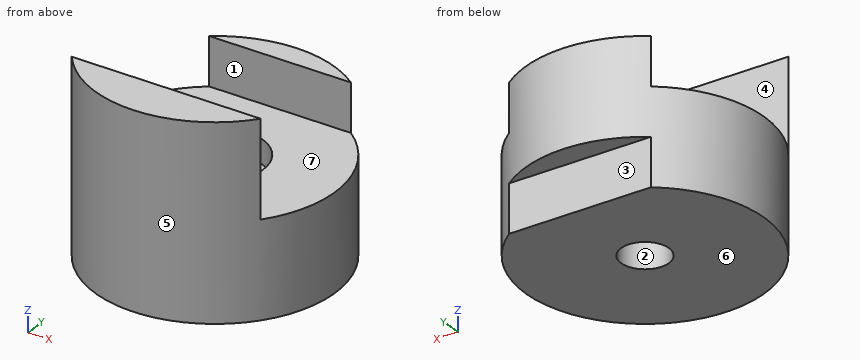
```python
from build123d import *

# Parameters (mm, degrees)
SKETCH1_R           = 5
SKETCH1_R_2         = 1
BOSS_EXTRUDE1_DEPTH = 8
SKETCH2_W           = 2
SKETCH2_H           = 1
CUT_EXTRUDE1_DEPTH  = 9
SKETCH3_R           = 2
CUT_EXTRUDE2_DEPTH  = 1


with BuildPart() as part:
    # Sketch1 → Boss-Extrude1 (new body)
    with BuildSketch(Plane.XY):
        Circle(SKETCH1_R)
        Circle(SKETCH1_R_2, mode=Mode.SUBTRACT)
    extrude(amount=BOSS_EXTRUDE1_DEPTH)

    # Sketch2 → Cut-Extrude1 (cut, symmetric)
    with BuildSketch(Plane(origin=(0, 0, 0), x_dir=(0, 0, -1), z_dir=(1, 0, 0))):
        Polygon((-8, -3), (-4, -3), (-4, 4), (-6, 4), (-6, 5), (-8, 5), align=None)
        with Locations((-1, 4.5)):
            Rectangle(SKETCH2_W, SKETCH2_H)
    extrude(amount=CUT_EXTRUDE1_DEPTH, both=True, mode=Mode.SUBTRACT)

    # Sketch3 → Cut-Extrude2 (cut)
    with BuildSketch(Plane.XY.offset(4)):
        Circle(SKETCH3_R)
    extrude(amount=-CUT_EXTRUDE2_DEPTH, mode=Mode.SUBTRACT)


solid = part.part
```
Build history of the part. All positions in model axes, mm. Face numbers are marked on the shaded views. A direction names the side the tool comes from. Coordinates: 2 decimals unless noted, no trailing zeros. Order: outer loops, then holes, each group sorted by start corner. A loop starts at its lowest first (then second) coordinate and runs counter-clockwise, first axis right, second up. Notation, with made-up numbers: (15.25, 19) -> (43.25, 19) arc R20 ccw to (43.25, 29) -> close; hole circle Ø3 at (-0.5, 40.25). An arc over 180 degrees is marked (long way). Answer in a Markdown table with one row per item. Add a question column.
Q1. Band-saw the part on C-C, the plane z = 5.5. List the corners of the cut face in (x, y).
Q2. Drop flat-ended pins along their axis: pin 1 (2 mm diameter, centred on x = -1, z = 5, fed in from -Y); pin 2 (1.2 mm diameter, centred on x = 0.5, y = 0, fed in from +Z); pin 3 (1.6 mm diameter, centred on x = -0.5, z = 1, fed in from +Y); pin 4 (3 mm diameter, centred on y = 3, z = 1.5, fed in from +X). Give the stop position or say it passes through.
Q3. Which spindle directions (+Z, -Z, +X, -X, +Y, -Y) get a long thin tool onto all of the face, cutting with end or side? Do the marked faces 1, 2 and 3. Say none if no direction does.
Q4. Band-saw the part on A-A, the plane x = 0. List the corners of the cut face in (y, z), then the cut area to 3 significant figures.
Q5. Band-saw the part on B-B, the plane y = 0. List the corners of the cut face in (x, z), then the cut area to 3 significant figures.
Q6. Mould opens along Y. For the marked faces 4, 5, 6 and 7 say: +Y half, -Y half, draft (parallel to the pull), parting line (faces both ways), or undercut.
Q7. Band-saw the part on D-D, the plane z = 0.75. List the corners of the cut face in (x, y), then the cut area to 3 significant figures.
Q8. Wall check: line 1 along Y through (x, z) = (0, 3.75); line 2 along Y through (x, z) = (0, 1.3); line 3 along X through (y, z) = (0, 1.1). Give the ranges that are in metal, low to high. Write a range as [from, to].
Answers follow:
| question | item | result |
|---|---|---|
| 1 | outline | (-4, -3) arc R5 ccw to (4, -3) -> close; (-3, 4) -> (3, 4) arc R5 ccw to start |
| 2 | pin 1 | y = -5 |
| 2 | pin 2 | z = 3 |
| 2 | pin 3 | y = 4 |
| 2 | pin 4 | x = 4.77 |
| 3 | face 1 | +Z, +X, -X |
| 3 | face 2 | +Z, -Z |
| 3 | face 3 | -Z, +X, -X, +Y |
| 4 | outline | (-5, 0) -> (-1, 0) -> (-1, 3) -> (-2, 3) -> (-2, 4) -> (-3, 4) -> (-3, 8) -> (-5, 8) -> close; (1, 0) -> (4, 0) -> (4, 2) -> (5, 2) -> (5, 6) -> (4, 6) -> (4, 4) -> (2, 4) -> (2, 3) -> (1, 3) -> close |
| 4 | area | 38.0 mm^2 |
| 5 | outline | (-5, 0) -> (-1, 0) -> (-1, 3) -> (-2, 3) -> (-2, 4) -> (-5, 4) -> close; (1, 0) -> (5, 0) -> (5, 4) -> (2, 4) -> (2, 3) -> (1, 3) -> close |
| 5 | area | 30.0 mm^2 |
| 6 | face 4 | undercut |
| 6 | face 5 | parting line |
| 6 | face 6 | draft |
| 6 | face 7 | undercut |
| 7 | outline | (-3, 4) arc R5 ccw (long way) to (3, 4) -> close; hole circle Ø2 at (0, 0) |
| 7 | area | 71.3 mm^2 |
| 8 | line 1 | [-5, -2], [2, 5] |
| 8 | line 2 | [-5, -1], [1, 4] |
| 8 | line 3 | [-5, -1], [1, 5] |
